from build123d import *

# Parameters (mm, degrees)
SKETCH1_W           = 0.92
SKETCH1_H           = 0.92
BOSS_EXTRUDE1_DEPTH = 3.5
SKETCH2_W           = 1
SKETCH2_H           = 1
BOSS_EXTRUDE2_DEPTH = 0.5


with BuildPart() as part:
    # Sketch1 → Boss-Extrude1 (new body, symmetric)
    with BuildSketch(Plane.XY):
        with Locations((0, 0.5)):
            Rectangle(SKETCH1_W, SKETCH1_H)
    extrude(amount=BOSS_EXTRUDE1_DEPTH, both=True)

    # Sketch2 → Boss-Extrude2 (add)
    with BuildSketch(Plane.XY.offset(3.5)):
        with Locations((0, 0.5)):
            Rectangle(SKETCH2_W, SKETCH2_H)
    boss_extrude2 = extrude(amount=BOSS_EXTRUDE2_DEPTH)

    # Mirror1: Boss-Extrude2 across plane
    add(boss_extrude2.mirror(Plane.XY))


solid = part.part
Design review of the part built by this model. Coordinates are the model's own, in mm. A direction names the side the tool comes from. Round coordinates to 2 decimals unless told otherwise and drop trailing zeros. Write each loop counter-clockwise with the first axis right and the second up, starting at its lowest first coordinate (ties: lowest second). Pieces come first, ordered by that corner, then holes. Notation, with made-up numbers: (54, -9) - (90, -9) arc R9 ccw to (90, 0) - close; hole circle Ø4 at (58.5, 37). An arc over 180 degrees is marked (long way). Return JSON: item names as keys, results as strings. Group by question number.
Item 1: Insertion check: P1, Ø0.5, axis at y = 0.5, z = 0, coming from the -X side; P2, Ø0.5, axis at y = 0.5, z = 1, coming from the +X side. Each pin has a flat end and moves straight along its axis. Give the tip position at first contact, or say it passes through.
Item 2: Machinability: for faces 4 (the face through (-0.46, 0.5, 0)), 5 (the face through (0, 0.96, 0)), 6 (the face through (0, 0.04, 0)), which of the approach directions +Z, -Z, +X, -X, +Y, -Y give a long, thin tool a straight path to every point of the face, cutting with its end or side? Answer none if there is none.
Item 3: We need section C-C on z = 2.5. Write out the cut boundary in (x, y), and give its area (3 significant figures).
Item 4: The part is to be moulded in two halves that separate along Z. For faces 1 (the face through (0.46, 0.5, 0)), 2 (the face through (0, 0.5, -4)), 3 (the face through (0, 0.5, 4)), say which applies: pulls with the +Z half, pulls with the -Z half, needs draft (parallel to the pull), parting line crosses it, or undercut.
Item 5: For probe 1 along Y at (x, z) = (0.15, 0.75); probe 2 along X at (y, z) = (0.2, -2.5), list the stretches that pass through material, from the lowest coordinate up. Write a range as [from, to].
Model answer:
{
 "1": {"P1": "stops at x = -0.46", "P2": "stops at x = 0.46"},
 "2": {"face 4": "-X, +Y, -Y", "face 5": "+X, -X, +Y", "face 6": "+X, -X, -Y"},
 "3": {"outline": "(-0.46, 0.04) - (0.46, 0.04) - (0.46, 0.96) - (-0.46, 0.96) - close", "area": "0.846 mm²"},
 "4": {"face 1": "undercut", "face 2": "pulls with the -Z half", "face 3": "pulls with the +Z half"},
 "5": {"probe 1": "y = [0.04, 0.96]", "probe 2": "x = [-0.46, 0.46]"}
}
